Geometry: see drawing. Coordinates: mm, zero at the bounding-box minimum. Round coordinates to 2 decimals unless told otherwise and drop trailing zeros. Write each loop counter-clockwise with the first axis right and the second up, starting at its lowest first coordinate (ties: lowest second). Pieces come first, ordered by that corner, then holes. Notation, with made-up numbers: M 75,-33.5 L 87,-33.5 A19 cw 87,-24.5 Z; hole C 70.5,43.25 d5. An arc over 180 degrees is marked long. Use a Markdown table: item, result.
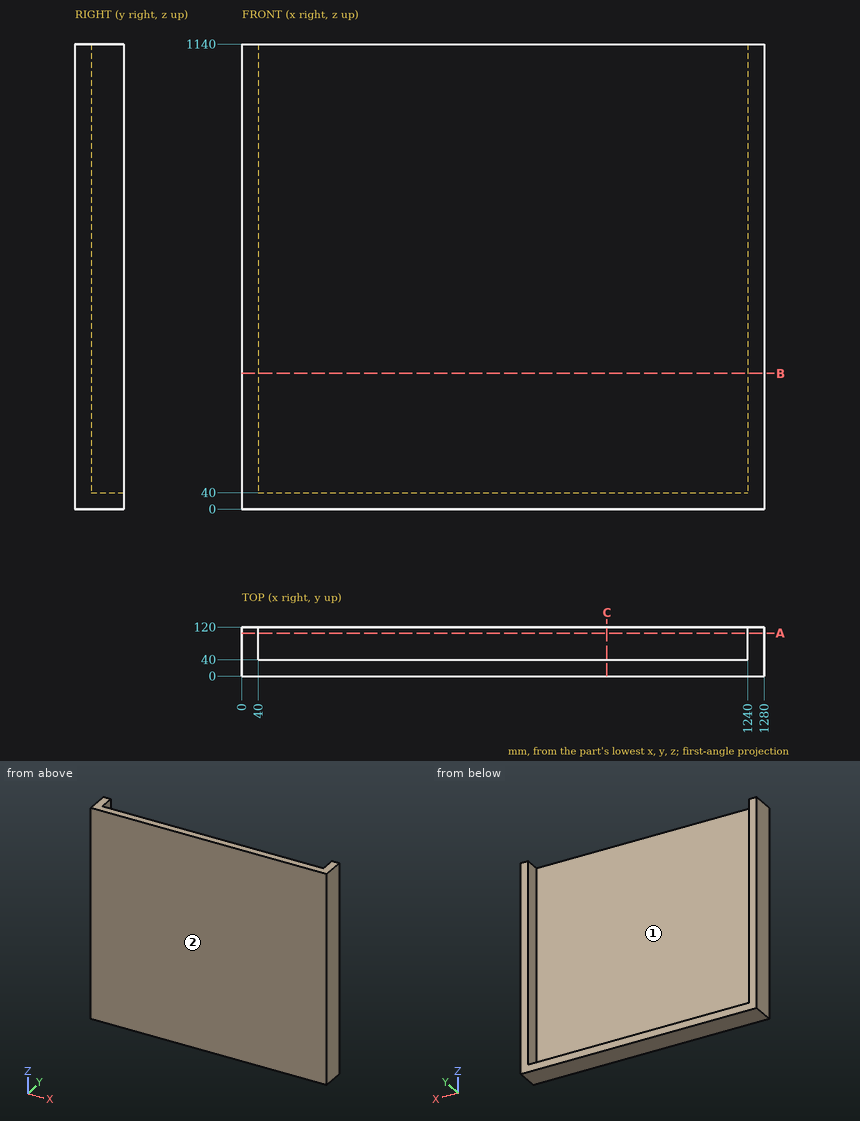
Q1. Section A-A on y = 105. Return loops of the section in (x, z), plus the area to 3 significant figures.
Results are:
| item | result |
|---|---|
| outline | M 0,0 L 1280,0 L 1280,1140 L 1240,1140 L 1240,40 L 40,40 L 40,1140 L 0,1140 Z |
| area | 139,000 mm^2 |
Q2. Section B-B on z = 332.5. Return loops of the section in (x, y).
Results are:
| item | result |
|---|---|
| outline | M 0,0 L 1280,0 L 1280,120 L 1240,120 L 1240,40 L 40,40 L 40,120 L 0,120 Z |
Q3. Line query: L1, parallel to X at y = 68, z = 484; L2, parallel to Y at x = 509.5, z = 93. Output: solid intervals per line, ascending.
Results are:
| item | result |
|---|---|
| L1 | 0 to 40, 1240 to 1280 |
| L2 | 0 to 40 |
Q4. Mould query, pull axis X, two halves, no side actions, for the marked faces 1 and 2. Classes: +X half, -X half, draft (parallel to the pull), parting line (faces both ways), or undercut.
Results are:
| item | result |
|---|---|
| face 1 | undercut |
| face 2 | draft |
Q5. First-contact query: pin 1 Ø1 at (x, y) = (728.5, 86) entering from +Z; pin 2 Ø1 at (x, z) = (396, 900.5) entering from +Y. Flat tips, straight axial feed; report the tip coordinate or a pass-through.
Results are:
| item | result |
|---|---|
| pin 1 | z = 40 |
| pin 2 | y = 40 |
Q6. Section C-C on x = 894.5. Return loops of the section in (y, z), plus the area to 3 significant figures.
Results are:
| item | result |
|---|---|
| outline | M 0,0 L 120,0 L 120,40 L 40,40 L 40,1140 L 0,1140 Z |
| area | 48,800 mm^2 |
